Geometry: final body of the model. Coordinates: model frame, mm. A direction names the side the tool comes from. Give positions to 0.01 mm unless a question says otherwise; leave off trailing zeros. Loops run counter-clockwise (first coordinate to the right, second up) from the corner with the lowest first, then second, coordinate; pieces in that order, holes last.
1. Section B-B, the plane y = -0.7. Output: boundary loops of the cut face in (x, z).
2. Section A-A, the plane z = -53. Output: boundary loops of the cut face in (x, y).
3. Material intervals for line 1 along Z through (x, y) = (11.5, -1.05); line 2 along X through (y, z) = (-0.9, -53.5); line 3 along Z through (x, y) = (-33, -1.35), sorted ascending.
4. First-contact query: P1, Ø0.6, axis at x = 3.5, y = -0.5, coming from the -Z side; P2, Ø1, axis at y = -1, z = -57, coming from the +X side; P3, Ø1, axis at y = -1, z = -58, coming from the -X side. Flat tips, straight axial feed; report the tip coordinate or a pass-through.
5. Section C-C, the plane x = 37.5. Output: boundary loops of the cut face in (y, z).
6. Draft query along Z for faces 6 (the face through (25.618, -1, -56)), 7 (the face through (3, -1, -9.378)), 8 (the face through (3, -1, -20.946)). Return one class per face: +Z half, -Z half, draft (parallel to the pull), parting line (faces both ways), or undercut.
7. Access query for faces 1 (the face through (-6.882, -1, -20)), 2 (the face through (-19.382, -1, -56)), 3 (the face through (43.118, -1, -30)), 4 (the face through (-32, -1, -51.378)), 5 (the face through (33.618, -1, -56)). Directions: +Z, -Z, +X, -X, +Y, -Y. A direction counts if a zero-diameter tool reaches every point of the face in a straight line with its end or side. Return the directions, or none.
from build123d import *

# Parameters (mm, degrees)
SKETCH_4_W               = 80
SKETCH_4_H               = 52
EXTRUDE_2_DEPTH          = 2
CUT_EXTRUDE_4_DEPTH      = 35
CUT_EXTRUDE_4_DEPTH_BACK = 32
SKETCH_5_W               = 9.5
SKETCH_5_H               = 10
CUT_EXTRUDE_5_DEPTH      = 54
CUT_EXTRUDE_5_DEPTH_BACK = 45
SKETCH_6_W               = 45
SKETCH_6_H               = 10
CUT_EXTRUDE_6_DEPTH      = 64
CUT_EXTRUDE_6_DEPTH_BACK = 67
SKETCH_7_W               = 9.5
SKETCH_7_H               = 10
CUT_EXTRUDE_7_DEPTH      = 30
CUT_EXTRUDE_7_DEPTH_BACK = 30
SKETCH_8_R               = 1.5
CHAMFER_1_SIZE           = 2
CUT_EXTRUDE_8_DEPTH      = 20
CUT_EXTRUDE_8_DEPTH_BACK = 33
SKETCH_9_R               = 1.5
CHAMFER_2_SIZE           = 2
SKETCH_10_W              = 20
SKETCH_10_H              = 2
CUT_EXTRUDE_9_DEPTH      = 2


with BuildPart() as part:
    # Эскиз4 → Бобышка-Вытянуть2 (new body)
    with BuildSketch(Plane(origin=(0, 0, 0), x_dir=(1, 0, 0), z_dir=(0, 1, 0))):
        with Locations((3.117803535, 35.377543141)):
            Rectangle(SKETCH_4_W, SKETCH_4_H)
    extrude(amount=-EXTRUDE_2_DEPTH)

    # Эскиз5 → Вырез-Вытянуть4 (cut, two sides: drawn at the far end of the back side and taken through both)
    with BuildSketch(Plane(origin=(0, 0, 0), x_dir=(1, 0, 0), z_dir=(0, 1, 0)).offset(-CUT_EXTRUDE_4_DEPTH_BACK)):
        with Locations((-32.132196465, 56.377543141)):
            Rectangle(SKETCH_5_W, SKETCH_5_H)
    extrude(amount=CUT_EXTRUDE_4_DEPTH + CUT_EXTRUDE_4_DEPTH_BACK, mode=Mode.SUBTRACT)

    # Эскиз6 → Вырез-Вытянуть5 (cut, two sides: drawn at the far end of the back side and taken through both)
    with BuildSketch(Plane(origin=(0, 0, 0), x_dir=(1, 0, 0), z_dir=(0, 1, 0)).offset(-CUT_EXTRUDE_5_DEPTH_BACK)):
        with Locations((3.117803535, 56.377543141)):
            Rectangle(SKETCH_6_W, SKETCH_6_H)
    extrude(amount=CUT_EXTRUDE_5_DEPTH + CUT_EXTRUDE_5_DEPTH_BACK, mode=Mode.SUBTRACT)

    # Эскиз7 → Вырез-Вытянуть6 (cut, two sides: drawn at the far end of the back side and taken through both)
    with BuildSketch(Plane(origin=(0, 0, 0), x_dir=(1, 0, 0), z_dir=(0, 1, 0)).offset(-CUT_EXTRUDE_6_DEPTH_BACK)):
        with Locations((38.367803535, 56.377543141)):
            Rectangle(SKETCH_7_W, SKETCH_7_H)
    extrude(amount=CUT_EXTRUDE_6_DEPTH + CUT_EXTRUDE_6_DEPTH_BACK, mode=Mode.SUBTRACT)

    # Эскиз8 → Вырез-Вытянуть7 (cut, two sides: drawn at the far end of the back side and taken through both)
    with BuildSketch(Plane(origin=(0, 0, 0), x_dir=(1, 0, 0), z_dir=(0, 1, 0)).offset(-CUT_EXTRUDE_7_DEPTH_BACK)):
        with Locations(Location((-23.382196465, 57.377543141, 0), (0, 0, 270))):
            Circle(SKETCH_8_R)
    extrude(amount=CUT_EXTRUDE_7_DEPTH + CUT_EXTRUDE_7_DEPTH_BACK, mode=Mode.SUBTRACT)

    # Фаска1
    chamfer_1_edges = [part.edges().sort_by_distance(p)[0] for p in [
        (-23.382196465, 0, -58.877543141),
    ]]
    chamfer(chamfer_1_edges, length=CHAMFER_1_SIZE - 0.0001)  # a hair under: the kernel refuses the full size

    # Эскиз9 → Вырез-Вытянуть8 (cut, two sides: drawn at the far end of the back side and taken through both)
    with BuildSketch(Plane(origin=(0, 0, 0), x_dir=(1, 0, 0), z_dir=(0, 1, 0)).offset(-CUT_EXTRUDE_8_DEPTH_BACK)):
        with Locations(Location((29.617803535, 57.377543141, 0), (0, 0, 270))):
            Circle(SKETCH_9_R)
    extrude(amount=CUT_EXTRUDE_8_DEPTH + CUT_EXTRUDE_8_DEPTH_BACK, mode=Mode.SUBTRACT)

    # Фаска2
    chamfer_2_edges = [part.edges().sort_by_distance(p)[0] for p in [
        (29.617803535, 0, -58.877543141),
    ]]
    chamfer(chamfer_2_edges, length=CHAMFER_2_SIZE - 0.0001)  # a hair under: the kernel refuses the full size

    # Эскиз10 → Вырез-Вытянуть9 (cut)
    with BuildSketch(Plane(origin=(0, 0, 0), x_dir=(1, 0, 0), z_dir=(0, 1, 0))):
        with Locations((3.117803535, 16.946236335)):
            Rectangle(SKETCH_10_W, SKETCH_10_H)
        with Locations((3.117803535, 19.946236335)):
            Rectangle(SKETCH_10_W, SKETCH_10_H)
    extrude(amount=-CUT_EXTRUDE_9_DEPTH, mode=Mode.SUBTRACT)


solid = part.part
Answers below:
1. outline: (-36.88, -51.38) - (-27.38, -51.38) - (-27.38, -61.38) - (-19.38, -61.38) - (-19.38, -51.38) - (25.62, -51.38) - (25.62, -61.38) - (33.62, -61.38) - (33.62, -51.38) - (43.12, -51.38) - (43.12, -9.38) - (-36.88, -9.38) - close; hole circle Ø5.6 at (-23.38, -57.38); hole (-6.88, -20.95) - (13.12, -20.95) - (13.12, -18.95) - (-6.88, -18.95) - close; hole (-6.88, -17.95) - (13.12, -17.95) - (13.12, -15.95) - (-6.88, -15.95) - close; hole circle Ø5.6 at (29.62, -57.38)
2. outline: (-27.38, -2) - (-19.38, -2) - (-19.38, 0) - (-27.38, 0) - close; (25.62, -2) - (33.62, -2) - (33.62, 0) - (25.62, 0) - close
3. line 1: z = -51.38 to -20.95, -18.95 to -17.95, -15.95 to -9.38
3. line 2: x = -27.38 to -19.38, 25.62 to 33.62
3. line 3: z = -51.38 to -9.38
4. P1: stops at z = -51.38
4. P2: stops at x = 33.62
4. P3: stops at x = -27.38
5. outline: (-2, -51.38) - (0, -51.38) - (0, -9.38) - (-2, -9.38) - close
6. face 6: draft
6. face 7: +Z half
6. face 8: undercut
7. face 1: +Y, -Y
7. face 2: -Z, +Y, -Y
7. face 3: +Z, -Z, +X, +Y, -Y
7. face 4: -Z, -X, +Y, -Y
7. face 5: -Z, +X, +Y, -Y
